from build123d import *

# Parameters (mm, degrees)
F0_W          = 21.9
F0_H          = 54.784943187
F2_DEPTH      = 13.95
F0_R          = 1.4
F3_DEPTH      = 2
F1_R          = 7.95
F4_DEPTH      = 27.3934715935
F4_DEPTH_BACK = 27.3934715935
F7_R          = 14.5
F7_R_2        = 12.5
F8_R          = 14.5
F8_R_2        = 12.5
F9_DEPTH      = 3
F10_T1_DEPTH  = 59.6298977105
F11_T1_DEPTH  = 72.9200798033
F12_SIZE      = 0.5


# Not quite as in the source:
# - a fillet or chamfer that OpenCascade refuses, or shapes differently, is made with other operations: its cross-section is extruded or revolved along the edge and cut away or added


with BuildPart() as f2:
    # F0 (on Top) → F2 (new body)
    with BuildSketch(Plane.XY):
        Rectangle(F0_W, F0_H)
    extrude(amount=F2_DEPTH)

    # F0 (on Top) → F3 (join)
    with BuildSketch(Plane.XY):
        with BuildLine():
            ThreePointArc((10.95, -27.3924715935), (24.4261642507, -16.5412363504), (29.5, 0))
            ThreePointArc((29.5, 0), (24.4261642507, 16.5412363504), (10.95, 27.3924715935))
            Line((10.95, 27.3924715935), (10.95, -27.3924715935))
        make_face()
        with Locations((20.9, -3)):
            Circle(F0_R, mode=Mode.SUBTRACT)
        with BuildLine():
            Line((-10.95, -27.3924715935), (-10.95, 27.3924715935))
            ThreePointArc((-10.95, 27.3924715935), (-29.5, 0), (-10.95, -27.3924715935))
        make_face()
        with Locations((-20.9, -3)):
            Circle(F0_R, mode=Mode.SUBTRACT)
    extrude(amount=F3_DEPTH)

    # F1 (on Front) → F4 (cut, two sides)
    with BuildSketch(Plane.XZ) as f4_sk:
        with Locations((0, 11.95)):
            Circle(F1_R)
    extrude(amount=-F4_DEPTH, mode=Mode.SUBTRACT)
    extrude(f4_sk.sketch, amount=F4_DEPTH_BACK, mode=Mode.SUBTRACT)

    # F7 (on offset) + F8 (on offset) → F9 (cut, symmetric)
    with BuildSketch(Plane.XZ.offset(16)):
        with Locations((0, 16.1)):
            Circle(F7_R)
        with Locations((0, 16.1)):
            Circle(F7_R_2, mode=Mode.SUBTRACT)
    with BuildSketch(Plane.XZ.offset(-16)):
        with Locations((0, 16.1)):
            Circle(F8_R)
        with Locations((0, 16.1)):
            Circle(F8_R_2, mode=Mode.SUBTRACT)
    extrude(amount=F9_DEPTH, both=True, mode=Mode.SUBTRACT)

    # F10: chamfer of 1 on 2 edges, made by hand

    # F10_s2 → F10_t1 (cut)
    with BuildSketch(Plane.XZ.offset(-29.8149488552)):
        with BuildLine():
            Line((-7.8447816072, 13.0377503134), (-8.6628360241, 13.9802075969))
            Line((-8.6628360241, 13.9802075969), (-8.6628360241, 14.0002075969))
            ThreePointArc((-8.6628360241, 14.0002075969), (-8.178576054, 13.97), (-7.694316084, 13.97))
            Line((-7.694316084, 13.97), (-7.6749593139, 13.9449685535))
            ThreePointArc((-7.6749593139, 13.9449685535), (-7.7779305741, 13.4955406772), (-7.8249803447, 13.0349378407))
            Line((-7.8249803447, 13.0349378407), (-7.8447816072, 13.0377503134))
        make_face()
        with BuildLine():
            Line((8.6628360241, 13.9802075969), (7.8447816072, 13.0377503134))
            Line((7.8447816072, 13.0377503134), (7.8249803447, 13.0349378407))
            ThreePointArc((7.8249803447, 13.0349378407), (7.7779305741, 13.4955406772), (7.6749593139, 13.9449685535))
            Line((7.6749593139, 13.9449685535), (7.694316084, 13.97))
            ThreePointArc((7.694316084, 13.97), (8.178576054, 13.97), (8.6628360241, 14.0002075969))
            Line((8.6628360241, 14.0002075969), (8.6628360241, 13.9802075969))
        make_face()
    extrude(amount=F10_T1_DEPTH, mode=Mode.SUBTRACT)

    # F11: fillet of radius 4 on 2 edges, made by hand

    # F11_s2 → F11_t1 (cut)
    with BuildSketch(Plane.XZ.offset(-36.4600399016)):
        with BuildLine():
            ThreePointArc((10.95, 10.3229726767), (10.3224222102, 12.4739651072), (8.6366157821, 13.95))
            Line((8.6366157821, 13.95), (10.95, 13.95))
            Line((10.95, 13.95), (10.95, 10.3229726767))
        make_face()
        with BuildLine():
            ThreePointArc((-10.95, 10.3229726767), (-10.3224222102, 12.4739651072), (-8.6366157821, 13.95))
            Line((-8.6366157821, 13.95), (-10.95, 13.95))
            Line((-10.95, 13.95), (-10.95, 10.3229726767))
        make_face()
    extrude(amount=F11_T1_DEPTH, mode=Mode.SUBTRACT)

    # F12
    f12_edges = [f2.edges().sort_by_distance(p)[0] for p in [
        (0, 27.392472, 4),
        (0, -27.392472, 4),
    ]]
    chamfer(f12_edges, length=F12_SIZE)


solid = f2.part
Input: part model. Units: mm. Frame: model coordinates. A direction names the side the tool comes from. Round coordinates to 2 decimals unless told otherwise and drop trailing zeros. Loops run counter-clockwise (first coordinate to the right, second up) from the corner with the lowest first, then second, coordinate; pieces in that order, holes last. Notation, with made-up numbers: (21, 36.5) -> (79, 36.5) arc R14 ccw to (79, 42.5) -> close; hole circle Ø1 at (-11.75, 40). An arc over 180 degrees is marked (long way). Answer as a JSON object with one key per item and string values. Group by question number.
1) Reachability of faces 4 (the flat face through (0, 13, 3)), 5 (the cylindrical face through (-29.496, 0.492, 0.986)), 6 (the flat face through (-18, 0, 2)) from +Z, -Z, +X, -X, +Y, -Y: full face, straight path, thin tool, end or side. Return the list, or none.
2) Section query C-C on y = -3. Output: boundary loops of the cut face in (x, z), plus the area to 3 significant figures.
3) Pin query (flat end, axial travel): pin 1 (4 mm diameter, centred on y = 5, z = 8.5, fed in from +X); pin 2 (8 mm diameter, centred on x = 9.5, y = -3.5, fed in from -Z); pin 3 (15 mm diameter, centred on x = -16, y = -7, fed in from +Z); pin 4 (4 mm diameter, centred on x = 1.5, z = 6, fed in from -Y). Return the tip coordinate at first contact, or that it passes through.
4) Section query A-A on z = 11.95. Output: boundary loops of the cut face in (x, y), plus the area to 3 significant figures.
5) Section query D-D on x = -20.9. Output: boundary loops of the cut face in (y, z), plus the area to 3 significant figures.
6) Draft query along Z for faces 1 (the flat face through (10.95, 0, 6)), 2 (the cylindrical face through (10.339, 0.383, 12.447)), 3 (the cylindrical face through (-0.2, 16, 3.6)). Return one class per face: +Z half, -Z half, draft (parallel to the pull), parting line (faces both ways), or undercut.
7) Section query B-B on x = 0. Output: boundary loops of the cut face in (y, z).
8) Ray query, L1, parallel to Z at x = 15, y = 5.5; L2, parallel to X at y = 5, z = 11.95; L3, parallel to X at y = -23, z = 5.75. Return the intervals inside material, ascending.
Reply:
{
 "1": {"face 4": "none", "face 5": "+Z, -Z, -X", "face 6": "+Z, -X, +Y, -Y"},
 "2": {"outline": "(-29.35, 0) -> (-22.3, 0) -> (-22.3, 2) -> (-29.35, 2) -> close; (-19.5, 0) -> (19.5, 0) -> (19.5, 2) -> (10.95, 2) -> (10.95, 10.32) arc R4 ccw to (8.64, 13.95) -> (7.87, 13.07) arc R7.95 cw (long way) to (-7.87, 13.07) -> (-8.64, 13.95) arc R4 ccw to (-10.95, 10.32) -> (-10.95, 2) -> (-19.5, 2) -> close; (22.3, 0) -> (29.35, 0) -> (29.35, 2) -> (22.3, 2) -> close", "area": "232 mm2"},
 "3": {"pin 1": "stops at x = 10.95", "pin 2": "stops at z = 0", "pin 3": "stops at z = 13.95", "pin 4": "stops at y = -27.08"},
 "4": {"outline": "(-10.6, -27.39) -> (-8.45, -27.39) -> (-7.95, -26.89) -> (-7.95, 26.89) -> (-8.45, 27.39) -> (-10.6, 27.39) -> close; (7.95, -26.89) -> (8.45, -27.39) -> (10.6, -27.39) -> (10.6, 27.39) -> (8.45, 27.39) -> (7.95, 26.89) -> close", "area": "290 mm2"},
 "5": {"outline": "(-20.82, 0) -> (-4.4, 0) -> (-4.4, 2) -> (-20.82, 2) -> close; (-1.6, 0) -> (20.82, 0) -> (20.82, 2) -> (-1.6, 2) -> close", "area": "77.7 mm2"},
 "6": {"face 1": "draft", "face 2": "+Z half", "face 3": "undercut"},
 "7": {"outline": "(-27.39, 0) -> (27.39, 0) -> (27.39, 3.5) -> (26.89, 4) -> (-26.89, 4) -> (-27.39, 3.5) -> close; hole (-19, 1.6) -> (-13, 1.6) -> (-13, 3.6) -> (-19, 3.6) -> close; hole (13, 1.6) -> (19, 1.6) -> (19, 3.6) -> (13, 3.6) -> close"},
 "8": {"L1": "z = 0 to 2", "L2": "x = -10.6 to -7.95, 7.95 to 10.6", "L3": "x = -10.95 to -4.98, 4.98 to 10.95"}
}
